from build123d import *

# Parameters (mm, degrees)
F1_R     = 11.05
F2_DEPTH = 8
F3_SIZE  = 0.25


with BuildPart() as f2:
    # F1 (on Top) → F2 (new body)
    with BuildSketch(Plane.XY):
        Polygon((30, -12.0666206261), (40.45, -6.033310313), (40.45, 6.033310313), (30, 12.0666206261), (27.6919892048, 10.7340899722), (19.55, 6.033310313), (19.55, -6.033310313), (27.6919892048, -10.7340899722), align=None)
        Polygon((21.55, 4.8786097747), (30, 9.7572195493), (38.45, 4.8786097747), (38.45, -4.8786097747), (30, -9.7572195493), (21.55, -4.8786097747), align=None, mode=Mode.SUBTRACT)
        Polygon((9.1506350946, -9.1506350946), (30, -12.0666206261), (27.6919892048, -10.7340899722), (9.6900481732, -8.2163442363), align=None)
        Polygon((27.6919892048, 10.7340899722), (30, 12.0666206261), (9.1506350946, 9.1506350946), (9.6900481732, 8.2163442363), align=None)
        Polygon((3.3493649054, -12.5), (9.1506350946, -9.1506350946), (9.6900481732, -8.2163442363), (12.5, -3.3493649054), (12.5, 3.3493649054), (9.6900481732, 8.2163442363), (9.1506350946, 9.1506350946), (3.3493649054, 12.5), (2.2705387483, 12.5), (-3.3493649054, 12.5), (-9.1506350946, 9.1506350946), (-11.9605869214, 4.2836557637), (-12.5, 3.3493649054), (-12.5, -3.3493649054), (-11.9605869214, -4.2836557637), (-9.1506350946, -9.1506350946), (-3.3493649054, -12.5), (2.2705387483, -12.5), align=None)
        Circle(F1_R, mode=Mode.SUBTRACT)
        Polygon((-4.55, -32.0140724266), (3.3493649054, -12.5), (2.2705387483, -12.5), (-4.55, -29.3490111188), align=None)
        Polygon((2.2705387483, 12.5), (3.3493649054, 12.5), (-4.55, 32.0140724266), (-4.55, 29.3490111188), align=None)
        Polygon((-15, -38.0473827396), (-4.55, -32.0140724266), (-4.55, -29.3490111188), (-4.55, -19.9474518005), (-15, -13.9141414875), (-23.1419892048, -18.6149211466), (-25.45, -19.9474518005), (-25.45, -32.0140724266), align=None)
        Polygon((-23.45, -21.1021523389), (-15, -16.2235425642), (-6.55, -21.1021523389), (-6.55, -30.8593718882), (-15, -35.7379816628), (-23.45, -30.8593718882), align=None, mode=Mode.SUBTRACT)
        Polygon((-4.55, 29.3490111188), (-4.55, 32.0140724266), (-15, 38.0473827396), (-25.45, 32.0140724266), (-25.45, 19.9474518005), (-23.1419892048, 18.6149211466), (-15, 13.9141414875), (-4.55, 19.9474518005), align=None)
        Polygon((-6.55, 30.8593718882), (-6.55, 21.1021523389), (-15, 16.2235425642), (-23.45, 21.1021523389), (-23.45, 30.8593718882), (-15, 35.7379816628), align=None, mode=Mode.SUBTRACT)
        Polygon((-23.1419892048, -18.6149211466), (-11.9605869214, -4.2836557637), (-12.5, -3.3493649054), (-25.45, -19.9474518005), align=None)
        Polygon((-12.5, 3.3493649054), (-11.9605869214, 4.2836557637), (-23.1419892048, 18.6149211466), (-25.45, 19.9474518005), align=None)
    extrude(amount=F2_DEPTH)

    # F3
    f3_edges = [f2.edges().sort_by_distance(p)[0] for p in [
        (35.225, -9.049965, 0),
        (40.45, 0, 0),
        (35.225, 9.049965, 0),
        (19.575318, 10.608628, 0),
        (6.25, 10.825318, 0),
        (-0.600318, 22.257036, 0),
        (-9.775, 35.030728, 0),
        (-20.225, 35.030728, 0),
        (-25.45, 25.980762, 0),
        (-18.975, 11.648408, 0),
        (-12.5, 0, 0),
        (-18.975, -11.648408, 0),
        (-25.45, -25.980762, 0),
        (-20.225, -35.030728, 0),
        (-9.775, -35.030728, 0),
        (-0.600318, -22.257036, 0),
        (6.25, -10.825318, 0),
        (19.575318, -10.608628, 0),
        (-19.070995, 16.264531, 0),
        (-9.775, 16.930797, 0),
        (-4.55, 24.648231, 0),
        (-1.139731, 20.924506, 0),
        (-0.539413, 12.5, 0),
        (-6.25, 10.825318, 0),
        (-10.555611, 6.717145, 0),
        (-17.551288, 11.449288, 0),
        (-10.555611, -6.717145, 0),
        (-6.25, -10.825318, 0),
        (-0.539413, -12.5, 0),
        (-1.139731, -20.924506, 0),
        (-4.55, -24.648231, 0),
        (-9.775, -16.930797, 0),
        (-19.070995, -16.264531, 0),
        (-17.551288, -11.449288, 0),
        (18.691019, 9.475217, 0),
        (23.620995, 8.3837, 0),
        (19.55, 0, 0),
        (23.620995, -8.3837, 0),
        (18.691019, -9.475217, 0),
        (11.095024, -5.782855, 0),
        (12.5, 0, 0),
        (11.095024, 5.782855, 0),
        (25.775, -7.317915, 0),
        (21.55, 0, 0),
        (25.775, 7.317915, 0),
        (34.225, 7.317915, 0),
        (38.45, 0, 0),
        (34.225, -7.317915, 0),
        (-11.05, 0, 0),
        (-23.45, -25.980762, 0),
        (-19.225, -18.662847, 0),
        (-10.775, -18.662847, 0),
        (-6.55, -25.980762, 0),
        (-10.775, -33.298677, 0),
        (-19.225, -33.298677, 0),
        (-19.225, 33.298677, 0),
        (-10.775, 33.298677, 0),
        (-6.55, 25.980762, 0),
        (-10.775, 18.662847, 0),
        (-19.225, 18.662847, 0),
        (-23.45, 25.980762, 0),
        (35.225, -9.049965, 8),
        (40.45, 0, 8),
        (35.225, 9.049965, 8),
        (19.575318, 10.608628, 8),
        (6.25, 10.825318, 8),
        (-0.600318, 22.257036, 8),
        (-9.775, 35.030728, 8),
        (-20.225, 35.030728, 8),
        (-25.45, 25.980762, 8),
        (-18.975, 11.648408, 8),
        (-12.5, 0, 8),
        (-18.975, -11.648408, 8),
        (-25.45, -25.980762, 8),
        (-20.225, -35.030728, 8),
        (-9.775, -35.030728, 8),
        (-0.600318, -22.257036, 8),
        (6.25, -10.825318, 8),
        (19.575318, -10.608628, 8),
        (-19.070995, 16.264531, 8),
        (-9.775, 16.930797, 8),
        (-4.55, 24.648231, 8),
        (-1.139731, 20.924506, 8),
        (-0.539413, 12.5, 8),
        (-6.25, 10.825318, 8),
        (-10.555611, 6.717145, 8),
        (-17.551288, 11.449288, 8),
        (-10.555611, -6.717145, 8),
        (-6.25, -10.825318, 8),
        (-0.539413, -12.5, 8),
        (-1.139731, -20.924506, 8),
        (-4.55, -24.648231, 8),
        (-9.775, -16.930797, 8),
        (-19.070995, -16.264531, 8),
        (-17.551288, -11.449288, 8),
        (18.691019, 9.475217, 8),
        (23.620995, 8.3837, 8),
        (19.55, 0, 8),
        (23.620995, -8.3837, 8),
        (18.691019, -9.475217, 8),
        (11.095024, -5.782855, 8),
        (12.5, 0, 8),
        (11.095024, 5.782855, 8),
        (25.775, -7.317915, 8),
        (21.55, 0, 8),
        (25.775, 7.317915, 8),
        (34.225, 7.317915, 8),
        (38.45, 0, 8),
        (34.225, -7.317915, 8),
        (-11.05, 0, 8),
        (-23.45, -25.980762, 8),
        (-19.225, -18.662847, 8),
        (-10.775, -18.662847, 8),
        (-6.55, -25.980762, 8),
        (-10.775, -33.298677, 8),
        (-19.225, -33.298677, 8),
        (-19.225, 33.298677, 8),
        (-10.775, 33.298677, 8),
        (-6.55, 25.980762, 8),
        (-10.775, 18.662847, 8),
        (-19.225, 18.662847, 8),
        (-23.45, 25.980762, 8),
    ]]
    chamfer(f3_edges, length=F3_SIZE)


solid = f2.part
Check sheet for the modelled part. Datum: model origin and axes. Units: mm. A direction names the side the tool comes from. Round coordinates to 2 decimals unless told otherwise and drop trailing zeros. Loops run counter-clockwise (first coordinate to the right, second up) from the corner with the lowest first, then second, coordinate; pieces in that order, holes last. Notation, with made-up numbers: (4.25, 59) - (50.25, 59) arc R19 cw to (50.25, 76) - close; hole circle Ø1 at (-11.5, 3.25). An arc over 180 degrees is marked (long way). Answer as CSV lines item,"result". Start each with the question number.
Item 1: Release check for a two-part mould opening along X. For faces 5 (the flat face through (-18.76, -11.58, 7.88)), 6 (the flat face through (19.697, 10.498, 0.123)) record: +X half, -X half, draft (parallel to the pull), parting line (faces both ways), or undercut.
Item 2: Section check D-D (x = 35). Record the boundary of the cut face in (y, z), and give its area (3 significant figures).
Item 3: Set-up check for faces 1 (the flat face through (-18.94, 11.809, 0.123)), 2 (the flat face through (34.284, -7.284, 3.948)), 3 (the flat face through (-10.518, 6.529, 0.123)), 4 (the flat face through (25.773, -7.463, 7.877)): record each of +Z, -Z, +X, -X, +Y, -Y from which the full face is reachable in a straight line by a thin tool's end or side.
Item 4: Section check A-A (y = 0). Count the separate pieces of the cut face and the enclosed holes in it, and give its area (3 significant figures).
Item 5: Depth check by flat-ended pin: P1, Ø2, axis at y = -24, z = 2, coming from the +X side; P2, Ø4, axis at y = 12.5, z = 6.5, coming from the +X side; P3, Ø1.5, axis at y = -27.5, z = 6.5, coming from the +X side. Enter the tip coordinate at first touch or a pass-through.
Item 6: Scan lines: line 1 (Y direction, x = -4, z = 6.25); line 2 (X direction, y = -22, z = 7); line 3 (Y direction, x = -5, z = 5.5). Record each from-to range of solid material in increasing order. Write a range as [from, to].
Report:
1,face 5,"-X half"
1,face 6,"undercut"
2,outline,"(-9.18, 0.25) - (-8.89, 0) - (-7.16, 0) - (-6.87, 0.25) - (-6.87, 7.75) - (-7.16, 8) - (-8.89, 8) - (-9.18, 7.75) - close; (6.87, 0.25) - (7.16, 0) - (8.89, 0) - (9.18, 0.25) - (9.18, 7.75) - (8.89, 8) - (7.16, 8) - (6.87, 7.75) - close"
2,area,"36.7 mm2"
3,face 1,"-Z, -X"
3,face 2,"+Z, -Z"
3,face 3,"-Z"
3,face 4,"+Z"
4,separate pieces,"4"
4,enclosed holes,"0"
4,area,"54.7 mm2"
5,P1,"stops at x = -0.9"
5,P2,"stops at x = 32.71"
5,P3,"stops at x = -2.42"
6,line 1,"y = [-30.66, -27.99], [-12.12, -10.3], [10.3, 12.12], [27.99, 30.66]"
6,line 2,"x = [-25.45, -23.45], [-6.55, -4.55], [-1.58, -0.5]"
6,line 3,"y = [-32.27, -19.69], [-11.55, -9.85], [9.85, 11.55], [19.69, 32.27]"
